Check sheet for the modelled part. Datum: model origin and axes. Units: mm. A direction names the side the tool comes from. Round coordinates to 2 decimals unless told otherwise and drop trailing zeros. Order: outer loops, then holes, each group sorted by start corner. A loop starts at its lowest first (then second) coordinate and runs counter-clockwise, first axis right, second up. Notation, with made-up numbers: (12.25, 13.25) -> (53.25, 13.25) arc R20 ccw to (53.25, 43.25) -> close; hole circle Ø8 at (-10.75, 61.5). An arc over 180 degrees is marked (long way). Use CSV: the item, a comma, the result in double quotes.
```python
from build123d import *

# Parameters (mm, degrees)
F1_DEPTH    = 15
F2_T1_DEPTH = 23.5358983849
F3_R        = 1.5
F4_DEPTH    = 10


# Not quite as in the source:
# - a fillet or chamfer that OpenCascade refuses, or shapes differently, is made with other operations: its cross-section is extruded or revolved along the edge and cut away or added


with BuildPart() as f1:
    # F0 (on Front) → F1 (new body)
    with BuildSketch(Plane.XZ):
        Polygon((-3.4063665882, 0), (-1.7031832941, 2.95), (1.7031832941, 2.95), (3.4063665882, 0), (1.7031832941, -2.95), (-1.7031832941, -2.95), (-2.3960036171, -4.15), (2.3960036171, -4.15), (4.7920072343, 0), (2.3960036171, 4.15), (-2.3960036171, 4.15), (-4.7920072343, 0), align=None)
    extrude(amount=F1_DEPTH)

    # F2: fillet of radius 3 on 2 edges, made by hand

    # F2_s2 → F2_t1 (cut)
    with BuildSketch(Plane.XZ.offset(-4.2679491924)):
        with BuildLine():
            ThreePointArc((-4.7920072343, 0), (-3.4978833466, 0.4749251787), (-2.5527767497, 1.4784609691))
            Line((-2.5527767497, 1.4784609691), (-3.4063665882, 0))
            Line((-3.4063665882, 0), (-4.7920072343, 0))
        make_face()
        with BuildLine():
            ThreePointArc((0.0039963829, -2.95), (-1.3376444036, -3.266718427), (-2.3960036171, -4.15))
            Line((-2.3960036171, -4.15), (-1.7031832941, -2.95))
            Line((-1.7031832941, -2.95), (0.0039963829, -2.95))
        make_face()
    extrude(amount=F2_T1_DEPTH, mode=Mode.SUBTRACT)

    # F3 (on face) → F4 (join)
    with BuildSketch(Plane(origin=(0, 0, -4.15), x_dir=(1, 0, 0), z_dir=(0, 0, -1))):
        with BuildLine():
            ThreePointArc((-2.3960036171, 7.5), (0, 5.1039963829), (2.3960036171, 7.5))
            ThreePointArc((2.3960036171, 7.5), (0, 9.8960036171), (-2.3960036171, 7.5))
        make_face()
        with Locations((0, 7.5)):
            Circle(F3_R, mode=Mode.SUBTRACT)
    extrude(amount=F4_DEPTH)


solid = f1.part
```
Q1. Sectioned sample at D-D, the plane x = 0.75. Enter the section's corners in (y, z).
Result sheet:
outline,"(-15, -4.15) -> (-9.78, -4.15) -> (-9.78, -14.15) -> (-8.8, -14.15) -> (-8.8, -4.15) -> (-6.2, -4.15) -> (-6.2, -14.15) -> (-5.22, -14.15) -> (-5.22, -4.15) -> (0, -4.15) -> (0, -2.95) -> (-15, -2.95) -> close; (-15, 2.95) -> (0, 2.95) -> (0, 4.15) -> (-15, 4.15) -> close"
Q2. Mould release check, pull along Y, two halves, no side actions. Record for faces 5 (the face through (3.2, -15, 0.9)), 6 (the face through (3.58, -7.4, -2.1)), 7 (the face through (0, -6, -9)), 8 (the face through (-0.312, -9.876, -9.08)): pulls with the +Y half, pulls with the -Y half, needs draft (parallel to the pull), parting line crosses it, or undercut.
Result sheet:
face 5,"pulls with the -Y half"
face 6,"needs draft"
face 7,"undercut"
face 8,"parting line crosses it"
Q3. Sectioned sample at A-A, the plane y = -4.25. Enter the section's corners in (x, z).
Result sheet:
outline,"(-4.79, 0) arc R3 ccw to (-2.55, 1.48) -> (-1.7, 2.95) -> (1.7, 2.95) -> (3.41, 0) -> (1.7, -2.95) -> (0, -2.95) arc R3 ccw to (-2.4, -4.15) -> (2.4, -4.15) -> (4.79, 0) -> (2.4, 4.15) -> (-2.4, 4.15) -> close"
Q4. Sectioned sample at B-B, the plane x = 3. Enter the section's corners in (y, z).
Result sheet:
outline,"(-15, -3.1) -> (0, -3.1) -> (0, -0.7) -> (-15, -0.7) -> close; (-15, 0.7) -> (0, 0.7) -> (0, 3.1) -> (-15, 3.1) -> close"
Q5. Access from +Z, -Z, +X, -X, +Y, -Y to the whole of each face (thin tool, end or side, straight path). Record for faces 1 (the face through (0, -7, 2.95)), 2 (the face through (2.57, -7.4, -1.45)), 3 (the face through (-3.514, -7.395, 0.464)), 4 (the face through (0, -7, -4.15)).
Result sheet:
face 1,"+Y, -Y"
face 2,"-X, +Y, -Y"
face 3,"-Z, +Y, -Y"
face 4,"-Z"
Q6. Sectioned sample at C-C, the plane z = -7.75. Enter the section's corners in (x, y), then the cut area to 3 significant figures.
Result sheet:
outline,"circle Ø4.79 at (0, -7.5); hole circle Ø3 at (0, -7.5)"
area,"11.0 mm^2"
Q7. Go/stop test with flat-tipped pins: pin 1 (2 mm diameter, centred on y = -13, z = -4.5, fed in from +X); pin 2 (3 mm diameter, centred on y = -7.5, z = -5.5, fed in from +X); pin 3 (1.5 mm diameter, centred on y = -4.5, z = 1.5, fed in from -X). Record where each tip stops, or that it passes through.
Result sheet:
pin 1,"stops at x = 2.77"
pin 2,"stops at x = 2.48"
pin 3,"stops at x = -4.36"
Q8. Scan lines: L1, parallel to Y at x = 0, z = -7; L2, parallel to X at y = -7.5, z = -8.5; L3, parallel to Z at x = -1.5, y = -13.5. Record each from-to range of solid material in increasing order.
Result sheet:
L1,"y = -9.9 to -9, -6 to -5.1"
L2,"x = -2.4 to -1.5, 1.5 to 2.4"
L3,"z = -4.15 to -3.35, 2.95 to 4.15"
